```python
from build123d import *

# Parameters (mm, degrees)
SKETCH1_W           = 40
SKETCH1_H           = 40
BOSS_EXTRUDE1_DEPTH = 40
CUT_EXTRUDE1_DEPTH  = 40
CUT_EXTRUDE4_DEPTH  = 20
CUT_EXTRUDE5_DEPTH  = 20
BOSS_EXTRUDE2_DEPTH = 20
CUT_EXTRUDE6_DEPTH  = 50


with BuildPart() as part:
    # Sketch1 → Boss-Extrude1 (new body)
    with BuildSketch(Plane.XY):
        with Locations((20, 20)):
            Rectangle(SKETCH1_W, SKETCH1_H)
    extrude(amount=BOSS_EXTRUDE1_DEPTH)

    # Sketch2 → Cut-Extrude1 (cut)
    with BuildSketch(Plane.XY.offset(40)):
        Polygon((0, 0), (20, 40), (0, 40), align=None)
    extrude(amount=-CUT_EXTRUDE1_DEPTH, mode=Mode.SUBTRACT)

    # Sketch7 → Cut-Extrude4 (cut)
    with BuildSketch(Plane.XY.offset(40)):
        Polygon((20, 40), (20, 0), (0, 0), align=None)
    extrude(amount=-CUT_EXTRUDE4_DEPTH, mode=Mode.SUBTRACT)

    # Sketch8 → Cut-Extrude5 (cut)
    with BuildSketch(Plane.XY.offset(20)):
        Polygon((20, 40), (0, 0), (20, 0), align=None)
    extrude(amount=-CUT_EXTRUDE5_DEPTH, mode=Mode.SUBTRACT)

    # Sketch9 → Boss-Extrude2 (add)
    with BuildSketch(Plane.ZY.offset(-20)):
        Polygon((0, 40), (40, 0), (0, 0), align=None)
    extrude(amount=BOSS_EXTRUDE2_DEPTH)

    # Sketch10 → Cut-Extrude6 (cut)
    with BuildSketch(Plane(origin=(0, 0, 0), x_dir=(-1, 0, 0), z_dir=(0, 0, -1))):
        Polygon((0, 0), (-20, 40), (0, 40), align=None)
    extrude(amount=-CUT_EXTRUDE6_DEPTH, mode=Mode.SUBTRACT)


solid = part.part
```
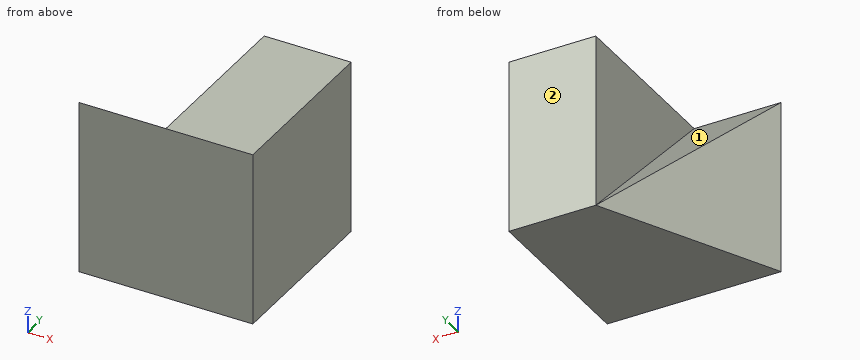
Check sheet for the modelled part. Datum: model origin and axes. Units: mm. Face numbers are marked on the shaded views. A direction names the side the tool comes from. Round coordinates to 2 decimals unless told otherwise and drop trailing zeros. Loops run counter-clockwise (first coordinate to the right, second up) from the corner with the lowest first, then second, coordinate; pieces in that order, holes last. Notation, with made-up numbers: (63.25, 48.25) -> (75.25, 48.25) arc R26 cw to (75.25, 86.25) -> close; hole circle Ø5 at (7.25, -10.75). An arc over 180 degrees is marked (long way). Write item = value, one per line. Start each with the question number.
1) Gauge pin test, flat end, axial feed: pin 1 Ø2 at (y, z) = (27.5, 17) entering from -X. Record the tip position at first contact, or that the pin passes through.
2) Sectioned sample at C-C, the plane x = 3. Record the cut outline in (y, z), plus the area to 3 significant figures.
3) Sectioned sample at B-B, the plane y = 15.5. Record the cut outline in (x, z).
4) Thickness scan on probe 1 along X at (y, z) = (21, 25); probe 2 along X at (y, z) = (3, 7); probe 3 along Z at (x, y) = (6, 6). Record the ranges inside material, lowest first.
5) Sectioned sample at A-A, the plane z = 27.5. Record the cut outline in (x, y), plus the area to 3 significant figures.
6) Set-up check for the marked faces 1 and 2: record each of +Z, -Z, +X, -X, +Y, -Y from which the full face is reachable in a straight line by a thin tool's end or side.
Results are:
q1.pin_1 = 20
q2.outline = (0, 0) -> (6, 0) -> (6, 34) -> (0, 40) -> close
q2.area = 222 mm^2
q3.outline = (7.75, 0) -> (40, 0) -> (40, 40) -> (20, 40) -> (20, 24.5) -> (7.75, 24.5) -> close
q4.probe_1 = 20 to 40
q4.probe_2 = 1.5 to 40
q4.probe_3 = 0 to 34
q5.outline = (0, 0) -> (40, 0) -> (40, 40) -> (20, 40) -> (20, 12.5) -> (6.25, 12.5) -> close
q5.area = 1,010 mm^2
q6.face_1 = +Z, -X, +Y
q6.face_2 = +Z, -Z, +X, -X, +Y
